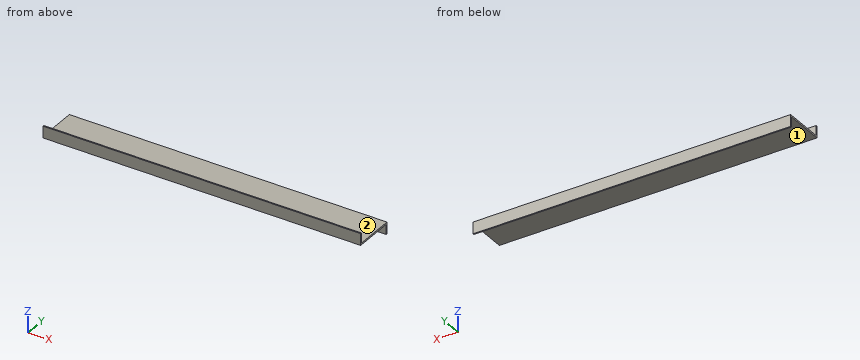
from build123d import *

# Parameters (mm, degrees)
SKETCH2_W           = 609.6
SKETCH2_H           = 78.74
BOSS_EXTRUDE1_DEPTH = 44.704
SKETCH4_W           = 19.05
SKETCH4_H           = 76.2
CUT_EXTRUDE1_DEPTH  = 617.287753583


with BuildPart() as part:
    # Sketch2 → Boss-Extrude1 (new body)
    with BuildSketch(Plane.XY):
        with Locations((304.8, 39.37)):
            Rectangle(SKETCH2_W, SKETCH2_H)
    extrude(amount=BOSS_EXTRUDE1_DEPTH)

    # Sketch4 → Cut-Extrude1 (cut, through all)
    with BuildSketch(Plane(origin=(609.6, 0, 0), x_dir=(0, 0, -1), z_dir=(1, 0, 0))):
        with Locations((-35.179, 40.64)):
            Rectangle(SKETCH4_W, SKETCH4_H)
        Polygon((0, 78.74), (-3.302, 78.74), (-3.302, 76.2), (-22.352, 76.2), (-22.352, 0), (0, 0), align=None)
    extrude(amount=-CUT_EXTRUDE1_DEPTH, mode=Mode.SUBTRACT)


solid = part.part
Verification items for the finished model (mm, model axes). Face numbers are marked on the shaded views. A direction names the side the tool comes from. Coordinates: 2 decimals unless noted, no trailing zeros. Order: outer loops, then holes, each group sorted by start corner. A loop starts at its lowest first (then second) coordinate and runs counter-clockwise, first axis right, second up. Notation, with made-up numbers: M 83.25,-36.5 L 139.25,-36.5 A19 ccw 139.25,-23.5 Z; hole C -28,66 d1. An arc over 180 degrees is marked long. One line per item, written item: value. Start each with the question number.
Item 1: Gauge pin test, flat ends, axial feed: pin 1 (5 mm diameter, centred on x = 220.5, z = 8, fed in from -Y); pin 2 (3 mm diameter, centred on x = 264, y = 55, fed in from +Z); pin 3 (1.5 mm diameter, centred on x = 253, z = 27, fed in from +Y). Record the tip position at first contact, or that the pin passes through.
Item 2: Scan lines: probe 1 along Z at (x, y) = (436, 54); probe 2 along Y at (x, z) = (135, 8.5); probe 3 along Y at (x, z) = (384, 42.5). Record each from-to range of solid material in increasing order.
Item 3: Sectioned sample at A-A (x = 466). Enter the section's corners in (y, z), then the cut area to 3 significant figures.
Item 4: Access from +Z, -Z, +X, -X, +Y, -Y to the whole of each face (thin tool, end or side, straight path). Record for the marked faces 1 and 2.
Item 5: Sectioned sample at C-C (y = 15). Enter the section's corners in (x, z), then the cut area to 3 significant figures.
Item 6: Sectioned sample at B-B (z = 39.5). Enter the section's corners in (x, y).
Conclusion:
1. pin 1: stops at y = 76.2
1. pin 2: stops at z = 25.65
1. pin 3: stops at y = 2.54
2. probe 1: z = 22.35 to 25.65
2. probe 2: y = 76.2 to 78.74
2. probe 3: y = 0 to 2.54
3. outline: M 0,22.35 L 76.2,22.35 L 76.2,3.3 L 78.74,3.3 L 78.74,25.65 L 2.54,25.65 L 2.54,44.7 L 0,44.7 Z
3. area: 357 mm^2
4. face 1: -Z, +X, -X, -Y
4. face 2: +Z, +X, -X, +Y
5. outline: M 0,22.35 L 609.6,22.35 L 609.6,25.65 L 0,25.65 Z
5. area: 2,010 mm^2
6. outline: M 0,0 L 609.6,0 L 609.6,2.54 L 0,2.54 Z
